from build123d import *

# Parameters (mm, degrees)
F2_DEPTH = 3


with BuildPart() as f2:
    # F1 (on offset) → F2 (new body)
    with BuildSketch(Plane.YZ.offset(-11.5)):
        Polygon((0, -4), (0, 0), (-11, 0), (-13.12132, -2.12132), (-39.12132, -2.12132), (-39.12132, -6.62132), (-11.964466, -6.62132), (-9.343146, -4), align=None)
    extrude(amount=-F2_DEPTH)


solid = f2.part
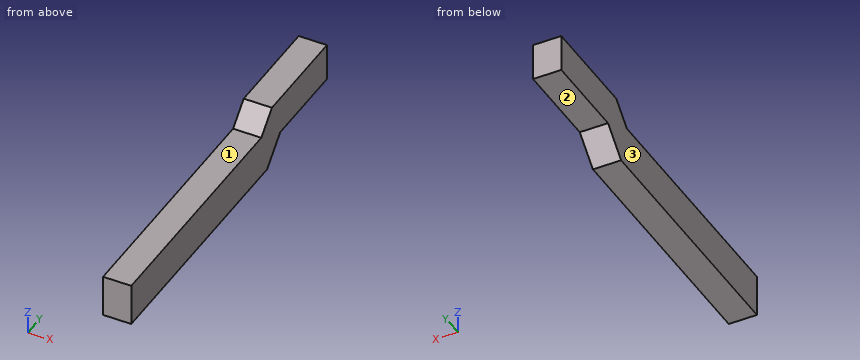
Could you check a few things on this model? Use its own coordinates, in mm. Face numbers are marked on the shaded views. A direction names the side the tool comes from. Give positions to 0.01 mm unless a question says otherwise; leave off trailing zeros. Write each loop counter-clockwise with the first axis right and the second up, starting at its lowest first coordinate (ties: lowest second). Pieces come first, ordered by that corner, then holes. Notation, with made-up numbers: (75, -36.5) - (104, -36.5) arc R14 ccw to (104, -26.5) - close; hole circle Ø5 at (1.5, -7). An arc over 180 degrees is marked (long way). Use CSV: the item, a comma, the result in double quotes. Start each with the question number.
Item 1: I'm going to push flat-ended pins straight in: pin 1 (1.5 mm diameter, centred on x = -13.5, y = -21, fed in from +Z); pin 2 (0.9 mm diameter, centred on x = -13.5, y = -4.5, fed in from -Z). Where does each tip first touch, or does it pass through?
Item 2: I want a section at C-C, the plane y = -6. Please give me the cut outline in (x, z), then the cut area to 3 significant figures.
Item 3: I want a section at A-A, the plane x = -13.7. Please give me the cut outline in (y, z).
Item 4: I want a section at B-B, the plane z = -1.75. Please give me the cut outline in (x, y), then the cut area to 4 significant figures.
Item 5: If I drill on line 1 along Z through (x, y) = (-12.45, -30); line 2 along Z through (x, y) = (-12.7, -5); line 3 along Y through (x, z) = (-13.5, -0.5), over which ranges is the centre line in solid material (lowest first)?
Item 6: For the marked faces 1, 2 and 3, which set-ups out of +Z, -Z, +X, -X, +Y, -Y let a thin tool reach every point of the face, with its end or its side?
Findings:
1,pin 1,"stops at z = -2.12"
1,pin 2,"stops at z = -4"
2,outline,"(-14.5, -4) - (-11.5, -4) - (-11.5, 0) - (-14.5, 0) - close"
2,area,"12.0 mm2"
3,outline,"(-39.12, -6.62) - (-11.96, -6.62) - (-9.34, -4) - (0, -4) - (0, 0) - (-11, 0) - (-13.12, -2.12) - (-39.12, -2.12) - close"
4,outline,"(-14.5, -12.75) - (-11.5, -12.75) - (-11.5, 0) - (-14.5, 0) - close"
4,area,"38.25 mm2"
5,line 1,"z = -6.62 to -2.12"
5,line 2,"z = -4 to 0"
5,line 3,"y = -11.5 to 0"
6,face 1,"+Z, +X, -X, -Y"
6,face 2,"-Z, +X, -X, +Y"
6,face 3,"+Z, -Z, -X, +Y, -Y"
